Could you check a few things on this model? Use its own coordinates, in mm. Face numbers are marked on the shaded views. A direction names the side the tool comes from. Give positions to 0.01 mm unless a question says otherwise; leave off trailing zeros. Loops run counter-clockwise (first coordinate to the right, second up) from the corner with the lowest first, then second, coordinate; pieces in that order, holes last.
1. Imagine slicing it at D-D (y = 0). List the corners of the cut face in (x, z) for me.
2. For P1, Ø3, axis at x = -6.5, z = -14, coming from the -Y side; P2, Ø5.5, axis at y = -3, z = -22, coming from the +X side; P3, Ø3, axis at x = -4, z = -14.5, coming from the +Y side, each with a flat end and sliding along its axis, tell me the tip position at first contact or that it passes through.
3. For the marked faces 1 and 2, which set-ups out of +Z, -Z, +X, -X, +Y, -Y let a thin tool reach every point of the face, with its end or its side?
4. I need wall thicknesses on line 1 along Y through (x, z) = (-4.3, 0); line 2 along X through (y, z) = (-0.75, -7.5); line 3 along Z through (x, y) = (-4.6, 0). Which ranges of each line are inside material? Lowest first, please.
5. Imagine slicing it at A-A (z = -32). List the corners of the cut face in (x, y) for me.
6. Imagine slicing it at C-C (z = 0). List the corners of the cut face in (x, y) for me, plus the area to 3 significant figures.
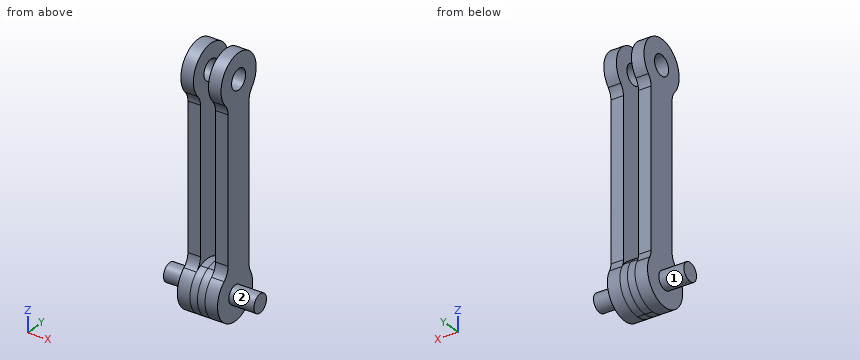
```python
from build123d import *
from build123d.topology import SkipClean

# Parameters (mm, degrees)
SKETCH_1_R               = 5
SKETCH_1_W               = 40
SKETCH_1_H               = 6
EXTRUDE_1_DEPTH          = 2.5
CUT_EXTRUDE_2_DEPTH      = 46.467021015
CUT_EXTRUDE_2_DEPTH_BACK = 46.467021015
SKETCH_1_3_R             = 2
FILLET_1_R               = 3
EXTRUDE_START            = -1.5
EXTRUDE_2_DEPTH          = 1.5
SKETCH_2_R               = 1.8
EXTRUDE_4_DEPTH          = 5
SKETCH_1_5_R             = 2
EXTRUDE_5_DEPTH          = 4


with BuildPart() as part:
    # Sketch 1 → Extrude 1 (new body)
    with BuildSketch(Plane(origin=(0, 0, 0), x_dir=(0, 0, -1), z_dir=(1, 0, 0))):
        Circle(SKETCH_1_R)
        with Locations((40, -1)):
            Circle(SKETCH_1_R)
        with Locations((20, 0)):
            Rectangle(SKETCH_1_W, SKETCH_1_H)
    extrude(amount=EXTRUDE_1_DEPTH)

    # Sketch 1_3 → Cut-Extrude 2 (cut, two sides: drawn at the far end of the back side and taken through both)
    with BuildSketch(Plane(origin=(0, 0, 0), x_dir=(0, 0, -1), z_dir=(1, 0, 0)).offset(-CUT_EXTRUDE_2_DEPTH_BACK)):
        Circle(SKETCH_1_3_R)
        with Locations((40, -1)):
            Circle(SKETCH_1_3_R)
    extrude(amount=CUT_EXTRUDE_2_DEPTH + CUT_EXTRUDE_2_DEPTH_BACK, mode=Mode.SUBTRACT)

    # Fillet 1
    fillet_1_edges = [part.edges().sort_by_distance(p)[0] for p in [
        (1.25, -3, -35.417424305),
        (1.25, 3, -37),
        (1.25, 3, -4),
        (1.25, -3, -4),
    ]]
    fillet(fillet_1_edges, radius=FILLET_1_R)

    # Sketch 1_4 → Extrude 2 (add)
    with SkipClean():  # the faces are left unmerged after this step: merging them gives an invalid solid
        with BuildSketch(Plane(origin=(0, 0, 0), x_dir=(0, 0, -1), z_dir=(1, 0, 0)).offset(EXTRUDE_START)):
            with BuildLine():
                ThreePointArc((37, 3), (35.16534763, 0.275200556), (35.417424305, -3))
                Line((35.417424305, -3), (40, -3))
                ThreePointArc((40, -3), (38, -1), (40, 1))
                Line((40, 1), (40, 3))
                Line((40, 3), (37, 3))
            make_face()
            with BuildLine():
                Line((40, -3), (35.417424305, -3))
                ThreePointArc((35.417424305, -3), (41.021548218, -5.894531565), (45, -1))
                ThreePointArc((45, -1), (42.236067977, 3.472135955), (37, 3))
                Line((37, 3), (40, 3))
                Line((40, 3), (40, 1))
                ThreePointArc((40, 1), (41.414213562, 0.414213562), (42, -1))
                ThreePointArc((42, -1), (41.414213562, -2.414213562), (40, -3))
            make_face()
        extrude(amount=EXTRUDE_2_DEPTH)



with BuildPart() as body_2:
    # Sketch 2 → Extrude 4 (new body)
    with BuildSketch(Plane(origin=(2.5, 0, 0), x_dir=(0, 0, -1), z_dir=(1, 0, 0))):
        with Locations((40, -1)):
            Circle(SKETCH_2_R)
    extrude(amount=EXTRUDE_4_DEPTH)


with BuildPart() as part_1:
    add(part.part)

    add(body_2.part)  # Extrude 5 merges body 2
    # Sketch 1_5 → Extrude 5 (add)
    with BuildSketch(Plane(origin=(0, 0, 0), x_dir=(0, 0, -1), z_dir=(1, 0, 0)).offset(EXTRUDE_START)):
        with Locations((40, -1)):
            Circle(SKETCH_1_5_R)
    extrude(amount=EXTRUDE_5_DEPTH)

    # Mirror 3: part across plane


with BuildPart() as part_2:
    add(part_1.part)
    add(part_1.part.mirror(Plane.ZY.offset(1.5)))


solid = part_2.part
```
Derived:
1. outline: (-10.5, -41.5) - (-5.5, -41.5) - (-5.5, -44.9) - (2.5, -44.9) - (2.5, -41.5) - (7.5, -41.5) - (7.5, -38.5) - (2.5, -38.5) - (2.5, -2) - (0, -2) - (0, -35.1) - (-3, -35.1) - (-3, -2) - (-5.5, -2) - (-5.5, -38.5) - (-10.5, -38.5) - close; (-5.5, 2) - (-3, 2) - (-3, 5) - (-5.5, 5) - close; (0, 2) - (2.5, 2) - (2.5, 5) - (0, 5) - close
2. P1: stops at y = -3
2. P2: stops at x = 2.5
2. P3: stops at y = 3
3. face 1: -X
3. face 2: +X
4. line 1: y = -5 to -2, 2 to 5
4. line 2: x = -5.5 to -3, 0 to 2.5
4. line 3: z = -44.9 to -2, 2 to 5
5. outline: (-5.5, -3) - (-3, -3) - (-3, 3) - (-5.5, 3) - close; (0, -3) - (2.5, -3) - (2.5, 3) - (0, 3) - close
6. outline: (-5.5, -5) - (-3, -5) - (-3, -2) - (-5.5, -2) - close; (-5.5, 2) - (-3, 2) - (-3, 5) - (-5.5, 5) - close; (0, -5) - (2.5, -5) - (2.5, -2) - (0, -2) - close; (0, 2) - (2.5, 2) - (2.5, 5) - (0, 5) - close
6. area: 30.0 mm2
